Check sheet for the modelled part. Datum: model origin and axes. Units: mm. Give positions to 0.01 mm unless a question says otherwise; leave off trailing zeros. Order: outer loops, then holes, each group sorted by start corner. A loop starts at its lowest first (then second) coordinate and runs counter-clockwise, first axis right, second up. Notation, with made-up numbers: (-33.5, -39.75) - (1.5, -39.75) arc R12 ccw to (1.5, -29.75) - close; hole circle Ø9 at (74.5, 77). An arc over 180 degrees is marked (long way). Answer in a Markdown table with one row per item.
from build123d import *

# Parameters (mm, degrees)
F1_DEPTH = 78.74
F2_R     = 5.08
F3_SIZE  = 5.08


with BuildPart() as f1:
    # F0 (on Top) → F1 (new body)
    with BuildSketch(Plane.XY):
        with BuildLine():
            ThreePointArc((-23.742214, 39.193708), (-39.775667, 2.693222), (0, 0))
            ThreePointArc((0, 0), (13.695812, 35.084423), (-23.742214, 39.193708))
        make_face()
    extrude(amount=F1_DEPTH)

    # F2
    f2_edges = [f1.edges().sort_by_distance(p)[0] for p in [
        (-39.775667, 2.693222, 78.74),
        (13.695812, 35.084423, 78.74),
    ]]
    fillet(f2_edges, radius=F2_R)

    # F3
    f3_edges = [f1.edges().sort_by_distance(p)[0] for p in [
        (-39.775667, 2.693222, 0),
        (13.695812, 35.084423, 0),
    ]]
    chamfer(f3_edges, length=F3_SIZE)


solid = f1.part
(1) Cross-section at A-A, the plane z = 34. Record the cut outline in (x, y).
Geometry says:
| item | result |
|---|---|
| outline | (-23.74, 39.19) arc R24.36 ccw (long way) to (0, 0) arc R23.73 ccw (long way) to start |
(2) Gauge pin test, flat ends, axial feed: P1, Ø5, axis at x = 4.5, y = 7, coming from the -Z side; P2, Ø4, axis at x = 8.5, z = 63, coming from the -Y side; P3, Ø1.5, axis at y = 17.5, z = 20.5, coming from the -X side; P4, Ø3, axis at x = -14.5, z = 9.5, coming from the +Y side. Record the tip position at first contact, or that the pin passes through.
Geometry says:
| item | result |
|---|---|
| P1 | z = 0 |
| P2 | y = 3.01 |
| P3 | x = -43.26 |
| P4 | y = 45.64 |
(3) Thickness scan on L1, parallel to Z at x = -26, y = 36; L2, parallel to X at y = -0.5, z = 18.5; L3, parallel to X at y = 34, z = 35.5. Record the ranges inside material, lowest first.
Geometry says:
| item | result |
|---|---|
| L1 | 2.58 to 78.04 |
| L2 | -37.47 to -0.42 |
| L3 | -34.57 to 14.31 |
